from build123d import *

# Parameters (mm, degrees)
F0_W        = 50
F0_H        = 100
F0_W_2      = 44
F0_H_2      = 94
F1_DEPTH    = 2832
F2_T1_DEPTH = 568.4974851551
F3_T1_DEPTH = 568.4974851551


# Not quite as in the source:
# - a fillet or chamfer that OpenCascade refuses, or shapes differently, is made with other operations: its cross-section is extruded or revolved along the edge and cut away or added


with BuildPart() as f1:
    # F0 (on Top) → F1 (new body)
    with BuildSketch(Plane.XY):
        Rectangle(F0_W, F0_H)
        Rectangle(F0_W_2, F0_H_2, mode=Mode.SUBTRACT)
    extrude(amount=F1_DEPTH)

    # F2: chamfer of 100 x 42 on 1 edges, made by hand

    # F2_s2 → F2_t1 (cut)
    with BuildSketch(Plane.YZ.offset(-284.2487425775)):
        Polygon((50, 2790), (-50, 2832), (50, 2832), align=None)
    extrude(amount=F2_T1_DEPTH, mode=Mode.SUBTRACT)

    # F3: chamfer of 42 x 100 on 1 edges, made by hand

    # F3_s2 → F3_t1 (cut)
    with BuildSketch(Plane.YZ.offset(-284.2487425775)):
        Polygon((-50, 0), (50, 42), (50, 0), align=None)
    extrude(amount=F3_T1_DEPTH, mode=Mode.SUBTRACT)


solid = f1.part
The model under review builds one solid part; all positions refer to its coordinate system, in mm. A direction names the side the tool comes from. Round coordinates to 2 decimals unless told otherwise and drop trailing zeros. Loops run counter-clockwise (first coordinate to the right, second up) from the corner with the lowest first, then second, coordinate; pieces in that order, holes last. Notation, with made-up numbers: (67, -16.75) -> (103, -16.75) arc R31 cw to (103, 22.25) -> close; hole circle Ø11 at (0.5, 3.5). An arc over 180 degrees is marked (long way). Return JSON: item names as keys, results as strings.
(1) Add section B-B on x = -14. Write out the cut boundary in (y, z), plus the area to 3 significant figures.
Solved:
{"outline": "(-50, 0) -> (-47, 1.26) -> (-47, 2830.74) -> (-50, 2832) -> close; (47, 40.74) -> (50, 42) -> (50, 2790) -> (47, 2791.26) -> close", "area": "16,700 mm2"}
(2) For line 1 (X direction, y = 13.5, z = 628); line 2 (Y direction, x = 10, z = 2129), list the stretches that pass through material, from the lowest coordinate up.
Solved:
{"line 1": "-25 to -22, 22 to 25", "line 2": "-50 to -47, 47 to 50"}
(3) Add section A-A on y = -16.5. Write out the cut boundary in (x, z), plus the area to 3 significant figures.
Solved:
{"outline": "(-25, 14.07) -> (-22, 14.07) -> (-22, 2817.93) -> (-25, 2817.93) -> close; (22, 14.07) -> (25, 14.07) -> (25, 2817.93) -> (22, 2817.93) -> close", "area": "16,800 mm2"}
(4) For pin 1 (8 mm diameter, centred on x = 15.5, y = -31, fed in from +Z), flat-tipped, find the tip position at first contact; note if it passes through.
Solved:
{"pin 1": "through"}
(5) Add section C-C on z = 1414. Write out the cut boundary in (x, y), plus the area to 3 significant figures.
Solved:
{"outline": "(-25, -50) -> (25, -50) -> (25, 50) -> (-25, 50) -> close; hole (-22, -47) -> (22, -47) -> (22, 47) -> (-22, 47) -> close", "area": "864 mm2"}
(6) For faces 4 (the flat face through (0, -50, 1396)), 5 (the flat face through (0, -47, 1396)), list the 3-axis set-ups (+Z, -Z, +X, -X, +Y, -Y) from which the entire face can be reached by the end or side of a thin tool; tool diameter is ignored.
Solved:
{"face 4": "+Z, -Z, +X, -X, -Y", "face 5": "+Z, -Z"}
(7) The part is to be moulded in two halves that separate along Y. For faces 1 (the flat face through (24, 0, 2811)), 2 (the flat face through (22, -1, 1396)), 3 (the flat face through (-25, -1, 1396)), say which applies: released by +Y, released by -Y, zero draft, split by the parting line, or undercut.
Solved:
{"face 1": "released by +Y", "face 2": "undercut", "face 3": "zero draft"}
